```python
from build123d import *

# Parameters (mm, degrees)
F1_DEPTH = 63.5
F3_DEPTH = 25.4
F5_DEPTH = 25.4
F7_DEPTH = 25.4


with BuildPart() as f1:
    # F0 (on Top) → F1 (new body)
    with BuildSketch(Plane.XY):
        Polygon((31.054489, 67.379584), (-45.145511, 67.379584), (-45.145511, 29.279584), (-19.745511, 29.279584), (-19.745511, -21.520416), (5.654489, -21.520416), (5.654489, 29.279584), (31.054489, 29.279584), align=None)
    extrude(amount=F1_DEPTH)

    # F2 (on face) → F3 (join)
    with BuildSketch(Plane.YZ.offset(5.654489)):
        Polygon((29.279584, 0), (29.279584, 63.5), (-21.520416, 0), align=None)
    extrude(amount=F3_DEPTH)

    # F4 (on face) → F5 (join)
    with BuildSketch(Plane.YZ.offset(5.654489)):
        Polygon((-21.520416, 0.954785), (-21.520416, 63.5), (-73.614173, 0), align=None)
    extrude(amount=-F5_DEPTH)

    # F6 (on face) → F7 (join)
    with BuildSketch(Plane(origin=(-19.745511, 0, 0), x_dir=(0, -1, 0), z_dir=(-1, 0, 0))):
        Polygon((21.520416, 0), (-29.279584, 63.5), (-29.279584, 0), align=None)
    extrude(amount=F7_DEPTH)


solid = f1.part
```
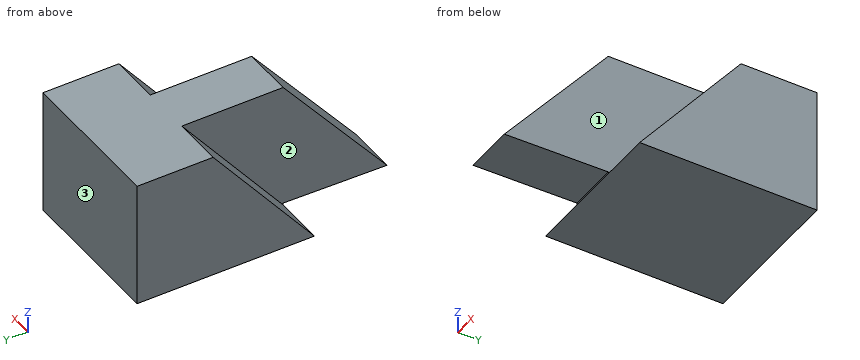
Geometry: final body of the model. Coordinates: model frame, mm. Face numbers are marked on the shaded views. A direction names the side the tool comes from. Round coordinates to 2 decimals unless told otherwise and drop trailing zeros. Write each loop counter-clockwise with the first axis right and the second up, starting at its lowest first coordinate (ties: lowest second). Pieces come first, ordered by that corner, then holes. Notation, with made-up numbers: M 68.5,85.5 L 114.5,85.5 A23 cw 114.5,103.5 Z; hole C 87,78 d8. An arc over 180 degrees is marked long. Answer in a Markdown table with one row per item. Add a question column.
(1) Reachability of the marked faces 1, 2 and 3 from +Z, -Z, +X, -X, +Y, -Y: full face, straight path, thin tool, end or side. Return the list, or none.
(2) Ray query, L1, parallel to X at y = -51.5, z = 19; L2, parallel to Y at x = 13.5, z = 13; L3, parallel to Y at x = -20, z = 29. Return the intervals inside material, ascending.
(3) Cut plane C-C, the plane z = 59. Return the cut outline in (x, y).
(4) Cut plane B-B, the plane x = -15.5. Return the cut outline in (y, z), then the cut area to 3 significant figures.
(5) Cut plane A-A, the plane y = 8. Return the cut outline in (x, z).
(6) Contact query for flat-ended pins moving along their axis: pin 1 (19 mm diameter, centred on y = -33, z = 30.5, fed in from -X); pin 2 (1.5 mm diameter, centred on x = -24, z = 48.5, fed in from -Y); pin 3 (5 mm diameter, centred on x = -9, y = -47, fed in from +Z); pin 4 (8 mm diameter, centred on x = 11.5, y = -44, fed in from -Z). Output: stop coordinate, or through.
(7) Cut plane D-D, the plane y = -49.5. Return the cut outline in (x, z), then the cut area to 3 significant figures.
Established:
| question | item | result |
|---|---|---|
| 1 | face 1 | +Z, +X, -Y |
| 1 | face 2 | +Z, -X, -Y |
| 1 | face 3 | +Z, -Z, +X, -X, +Y |
| 2 | L1 | -19.75 to 5.65 |
| 2 | L2 | -11.12 to 67.38 |
| 2 | L3 | 1.68 to 67.38 |
| 3 | outline | M -45.15,25.68 L -19.75,25.68 L -19.75,-25.21 L 5.65,-25.21 L 5.65,25.68 L 31.05,25.68 L 31.05,67.38 L -45.15,67.38 Z |
| 4 | outline | M -73.61,0 L -21.52,0.95 L -21.52,0 L 67.38,0 L 67.38,63.5 L -21.52,63.5 Z |
| 4 | area | 7,270 mm² |
| 5 | outline | M -45.15,0 L 31.05,0 L 31.05,36.9 L 5.65,36.9 L 5.65,63.5 L -19.75,63.5 L -19.75,36.9 L -45.15,36.9 Z |
| 6 | pin 1 | x = -19.75 |
| 6 | pin 2 | y = 16.68 |
| 6 | pin 3 | z = 35.49 |
| 6 | pin 4 | through |
| 7 | outline | M -19.75,0.44 L 5.65,0.44 L 5.65,29.39 L -19.75,29.39 Z |
| 7 | area | 735 mm² |
